Geometry check sheet. Reference: the model listing, model coordinates, mm. A direction names the side the tool comes from. Round coordinates to 2 decimals unless told otherwise and drop trailing zeros. Loops run counter-clockwise (first coordinate to the right, second up) from the corner with the lowest first, then second, coordinate; pieces in that order, holes last. Notation, with made-up numbers: M 55,71 L 81,71 A9 cw 81,76 Z; hole C 25,63 d8. An arc over 180 degrees is marked long. Use one line per item in the form item = value. Start each with the question number.
1. Cross-section at B-B (z = -183.5). Record the boundary of the cut face in (x, y), then the cut area to 3 significant figures.
2. Material ranges on line 1 (Z direction, x = 0.95, y = 158.5); line 2 (Y direction, x = -1.6, z = -144); line 3 (Y direction, x = 2, z = -215), recorded low to high.
3. Draft check along Z on faces 1 (the flat face through (0.038, 419.253, -221.85)), 2 (the flat face through (0.04, 390.15, -234.46)), 3 (the flat face through (2.75, 198, -228)). Enter one of: pulls with the +Z half, pulls with the -Z half, needs draft (parallel to the pull), parting line crosses it, or undercut.
4. Cross-section at A-A (y = 94). Record the boundary of the cut face in (x, z).
5. Cross-section at D-D (z = -377.5). Record the boundary of the cut face in (x, y), then the cut area to 3 significant figures.
6. Set-up check for faces 4 (the flat face through (-2.75, 198, -228)), 5 (the flat face through (0.04, 402.85, -229.78)): record each of +Z, -Z, +X, -X, +Y, -Y from which the full face is reachable in a straight line by a thin tool's end or side.
7. Go/stop test with flat-tipped pins: pin 1 (1.6 mm diameter, centred on x = 1, y = 333, fed in from +Z); pin 2 (3 mm diameter, centred on x = -0.5, z = -165.5, fed in from +Y); pin 3 (1 mm diameter, centred on x = -2, z = -262.5, fed in from +Y); pin 4 (3 mm diameter, centred on x = -0.5, z = -16.5, fed in from +Y). Record where each tip stops, or that it passes through.
8. Cross-section at C-C (x = -1.45). Record the boundary of the cut face in (y, z), then the cut area to 3 significant figures.
```python
from build123d import *

# Parameters (mm, degrees)
CROQUIS1_W              = 304.8
CROQUIS1_H              = 5.5
CROQUIS1_W_2            = 5.5
CROQUIS1_H_2            = 355.6
CROQUIS1_H_3            = 254
SALIENTE_EXTRUIR1_DEPTH = 2.75


with BuildPart() as part:
    # Croquis1 → Saliente-Extruir1 (new, symmetric)
    with BuildSketch(Plane(origin=(0, 0, 0), x_dir=(0, 0, -1), z_dir=(1, 0, 0))):
        Polygon((450, 0), (0, 0), (0, 500), (450, 336.21339458), align=None)
        Polygon((65.045304049, 462.810387737), (399.2, 341.18802477), (399.2, 330.18802477), (65.045304049, 451.810387737), align=None, mode=Mode.SUBTRACT)
        with Locations((208.28, 15.45)):
            Rectangle(CROQUIS1_W, CROQUIS1_H, mode=Mode.SUBTRACT)
        with Locations((15.45, 247.65)):
            Rectangle(CROQUIS1_W_2, CROQUIS1_H_2, mode=Mode.SUBTRACT)
        with Locations((434.55, 177.8)):
            Rectangle(CROQUIS1_W_2, CROQUIS1_H_3, mode=Mode.SUBTRACT)
    extrude(amount=SALIENTE_EXTRUIR1_DEPTH, both=True)


solid = part.part
```
Reported:
q1.outline = M -2.75,0 L 2.75,0 L 2.75,12.7 L -2.75,12.7 Z; M -2.75,18.2 L 2.75,18.2 L 2.75,408.7 L -2.75,408.7 Z; M -2.75,419.7 L 2.75,419.7 L 2.75,433.21 L -2.75,433.21 Z
q1.area = 2,290 mm²
q2.line_1 = -450 to -437.3, -431.8 to -18.2, -12.7 to 0
q2.line_2 = 0 to 12.7, 18.2 to 423.07, 434.07 to 447.59
q2.line_3 = 0 to 12.7, 18.2 to 397.23, 408.23 to 421.75
q3.face_1 = pulls with the -Z half
q3.face_2 = undercut
q3.face_3 = needs draft
q4.outline = M -2.75,-450 L 2.75,-450 L 2.75,-437.3 L -2.75,-437.3 Z; M -2.75,-431.8 L 2.75,-431.8 L 2.75,-18.2 L -2.75,-18.2 Z; M -2.75,-12.7 L 2.75,-12.7 L 2.75,0 L -2.75,0 Z
q5.outline = M -2.75,0 L 2.75,0 L 2.75,338.09 L -2.75,338.09 Z; M -2.75,349.09 L 2.75,349.09 L 2.75,362.6 L -2.75,362.6 Z
q5.area = 1,930 mm²
q6.face_4 = +Z, -Z, -X, +Y, -Y
q6.face_5 = +X, -X
q7.pin_1 = 0
q7.pin_2 = 440.31
q7.pin_3 = 404.64
q7.pin_4 = 494.54
q8.outline = M 0,-450 L 336.21,-450 L 500,0 L 0,0 Z; hole M 12.7,-360.68 L 18.2,-360.68 L 18.2,-55.88 L 12.7,-55.88 Z; hole M 50.8,-437.3 L 304.8,-437.3 L 304.8,-431.8 L 50.8,-431.8 Z; hole M 69.85,-18.2 L 425.45,-18.2 L 425.45,-12.7 L 69.85,-12.7 Z; hole M 330.19,-399.2 L 341.19,-399.2 L 462.81,-65.05 L 451.81,-65.05 Z
q8.area = 179,000 mm²
